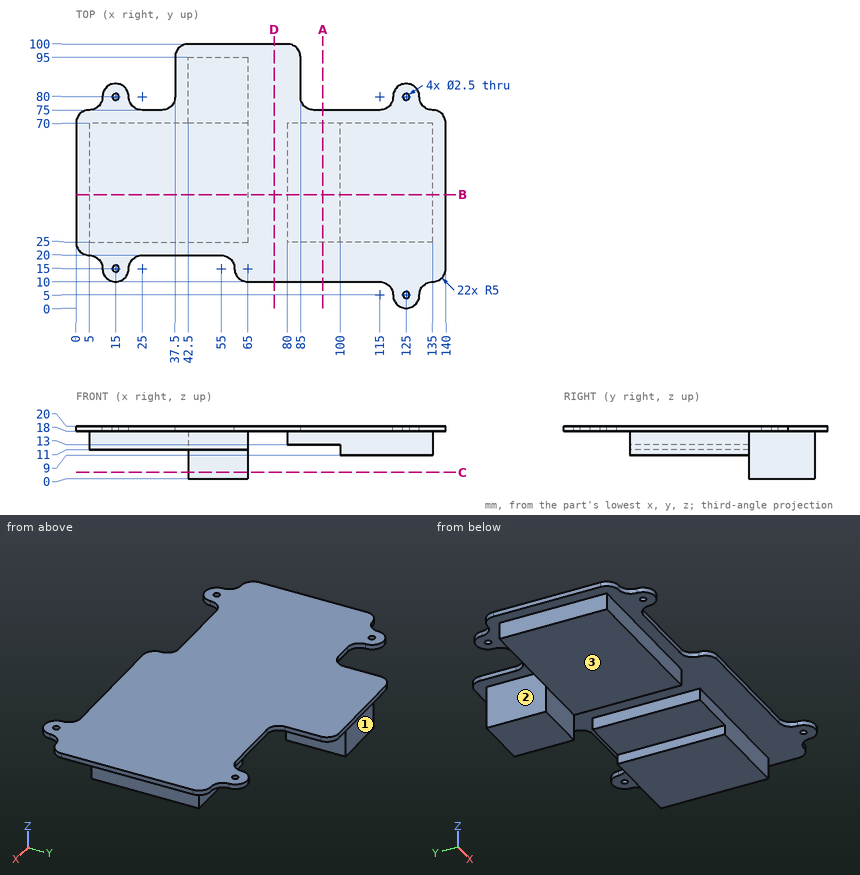
Print and shaded views of the part. All mm, measured from the part's lowest x, y and z. A direction names the side the tool comes from. Coordinates: 2 decimals unless noted, no trailing zeros. Loops run counter-clockwise (first coordinate to the right, second up) from the corner with the lowest first, then second, coordinate; pieces in that order, holes last. Notation, with made-up numbers: (67, 35) -> (79, 35) arc R19 ccw to (79, 65) -> close; hole circle Ø4 at (-2, 77). An arc over 180 degrees is marked (long way). Use a Markdown table: item, result. Add a question column.
Item 1: Which spindle directions (+Z, -Z, +X, -X, +Y, -Y) get a long thin tool onto all of the face, cutting with end or side? Do the marked faces 1, 2 and 3. Say none if no direction does.
Item 2: Band-saw the part on C-C on z = 2.5. Write the cut outline in (x, y), plus the area to 4 significant figures.
Item 3: Band-saw the part on A-A on x = 93.5. Write the cut outline in (y, z), plus the area to 3 significant figures.
Item 4: Flat gauge pins, fed straight in: P1, Ø1.5, axis at x = 15, y = 80, coming from the +Z side; P2, Ø8, axis at y = 27, z = 10, coming from the +X side; P3, Ø10, axis at x = 98.5, y = 42.5, coming from the -Z side; P4, Ø5, axis at x = 95, z = 17, coming from the +Y side. Where does each tip first touch, or does it go through?
Item 5: Probe probe 1 along Y at (x, z) = (125, 19.5); probe 2 along X at (y, z) = (80, 18.6); probe 3 along X at (y, z) = (31.5, 13.5). List the from-to ranges inside material, lowest first.
Item 6: Band-saw the part on B-B on y = 43. Write the cut outline in (x, z), plus the area to 4 significant figures.
Item 7: Band-saw the part on D-D on x = 75. Write the cut outline in (y, z), plus the area to 3 significant figures.
Geometry says:
| question | item | result |
|---|---|---|
| 1 | face 1 | -Z, +X, -X, +Y |
| 1 | face 2 | -Z, -X, +Y |
| 1 | face 3 | -Z, -X, -Y |
| 2 | outline | (42.5, 70) -> (65, 70) -> (65, 95) -> (42.5, 95) -> close |
| 2 | area | 562.5 mm² |
| 3 | outline | (10, 18) -> (25, 18) -> (25, 13) -> (70, 13) -> (70, 18) -> (75, 18) -> (75, 20) -> (10, 20) -> close |
| 3 | area | 355 mm² |
| 4 | P1 | through |
| 4 | P2 | x = 135 |
| 4 | P3 | z = 9 |
| 4 | P4 | y = 75 |
| 5 | probe 1 | 0 to 3.75, 6.25 to 78.75, 81.25 to 85 |
| 5 | probe 2 | 10 to 13.75, 16.25 to 20, 37.5 to 85, 120 to 123.75, 126.25 to 130 |
| 5 | probe 3 | 5 to 65, 80 to 135 |
| 6 | outline | (0, 18) -> (5, 18) -> (5, 11) -> (65, 11) -> (65, 18) -> (80, 18) -> (80, 13) -> (100, 13) -> (100, 9) -> (135, 9) -> (135, 18) -> (140, 18) -> (140, 20) -> (0, 20) -> close |
| 6 | area | 1,115 mm² |
| 7 | outline | (10, 18) -> (100, 18) -> (100, 20) -> (10, 20) -> close |
| 7 | area | 180 mm² |
